Verification items for the finished model (mm, model axes). Face numbers are marked on the shaded views. Round coordinates to 2 decimals unless told otherwise and drop trailing zeros. Loops run counter-clockwise (first coordinate to the right, second up) from the corner with the lowest first, then second, coordinate; pieces in that order, holes last. Notation, with made-up numbers: (-37.75, -6.75) - (13.25, -6.75) arc R16 cw to (13.25, 6.25) - close; hole circle Ø4 at (66.5, -24.5). An arc over 180 degrees is marked (long way). Use CSV: the item, a comma, the result in double quotes.
```python
from build123d import *

# Parameters (mm, degrees)
SKETCH1_R           = 2.637642313
SKETCH1_R_2         = 73
BOSS_EXTRUDE1_DEPTH = 20
SKETCH4_R           = 73
SKETCH4_R_2         = 52.25
BOSS_EXTRUDE2_DEPTH = 10
SKETCH5_R           = 73
BOSS_EXTRUDE3_DEPTH = 10


with BuildPart() as part:
    # Sketch1 → Boss-Extrude1 (new body)
    with BuildSketch(Plane(origin=(0, 0, 0), x_dir=(1, 0, 0), z_dir=(0, 1, 0))):
        with BuildLine():
            Line((77.460838348, -75.098177713), (77.460838348, 74.577424045))
            ThreePointArc((77.460838348, 74.577424045), (76.578174547, 76.708362964), (74.447235628, 77.591026765))
            Line((74.447235628, 77.591026765), (-75.22836613, 77.591026765))
            ThreePointArc((-75.22836613, 77.591026765), (-77.359305049, 76.708362964), (-78.24196885, 74.577424045))
            Line((-78.24196885, 74.577424045), (-78.24196885, -75.098177713))
            ThreePointArc((-78.24196885, -75.098177713), (-77.359305049, -77.229116632), (-75.22836613, -78.111780433))
            Line((-75.22836613, -78.111780433), (74.447235628, -78.111780433))
            ThreePointArc((74.447235628, -78.111780433), (76.578174547, -77.229116632), (77.460838348, -75.098177713))
        make_face()
        with Locations((-60.604326536, -60.47413812)):
            Circle(SKETCH1_R, mode=Mode.SUBTRACT)
        with Locations((-60.604326536, 59.953384452)):
            Circle(SKETCH1_R, mode=Mode.SUBTRACT)
        with Locations((59.823196035, 59.953384452)):
            Circle(SKETCH1_R, mode=Mode.SUBTRACT)
        with Locations((59.823196035, -60.47413812)):
            Circle(SKETCH1_R, mode=Mode.SUBTRACT)
        Circle(SKETCH1_R_2, mode=Mode.SUBTRACT)
    extrude(amount=BOSS_EXTRUDE1_DEPTH)

    # Sketch4 → Boss-Extrude2 (add)
    with BuildSketch(Plane(origin=(0, 20, 0), x_dir=(1, 0, 0), z_dir=(0, 1, 0))):
        Circle(SKETCH4_R)
        Circle(SKETCH4_R_2, mode=Mode.SUBTRACT)
    extrude(amount=-BOSS_EXTRUDE2_DEPTH)

    # Sketch5 → Boss-Extrude3 (add)
    with BuildSketch(Plane.XZ.offset(-10)):
        Circle(SKETCH5_R)
    extrude(amount=BOSS_EXTRUDE3_DEPTH)


solid = part.part
```
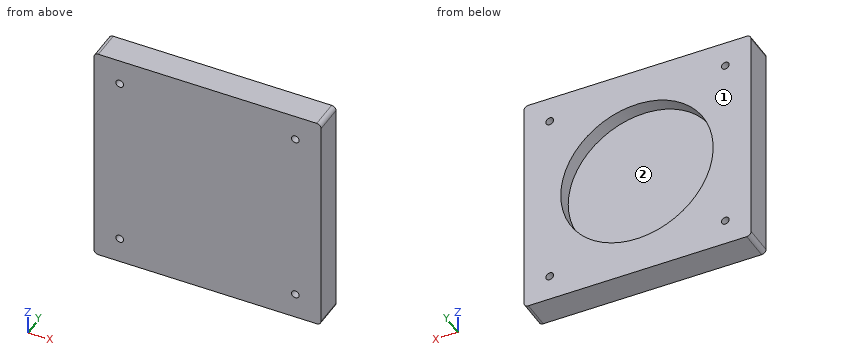
1) Thickness scan on probe 1 along X at (y, z) = (10.75, 0.5); probe 2 along Z at (x, y) = (0, 16.75); probe 3 along Z at (x, y) = (60.5, 18). Record the ranges inside material, lowest first. Write a range as [from, to].
Returned:
probe 1,"x = [-78.24, -52.25], [52.25, 77.46]"
probe 2,"z = [-77.59, -52.25], [52.25, 78.11]"
probe 3,"z = [-77.59, -62.5], [-57.4, 57.92], [63.02, 78.11]"
2) Cross-section at C-C, the plane y = 13.75. Record the cut outline in (x, z), then the cut area to 3 significant figures.
Returned:
outline,"(-78.24, -74.58) arc R3.01 ccw to (-75.23, -77.59) - (74.45, -77.59) arc R3.01 ccw to (77.46, -74.58) - (77.46, 75.1) arc R3.01 ccw to (74.45, 78.11) - (-75.23, 78.11) arc R3.01 ccw to (-78.24, 75.1) - close; hole circle Ø5.28 at (-60.6, -59.95); hole circle Ø5.28 at (-60.6, 60.47); hole circle Ø104.5 at (0, 0); hole circle Ø5.28 at (59.82, -59.95); hole circle Ø5.28 at (59.82, 60.47)"
area,"15,600 mm²"
3) Mould release check, pull along X, two halves, no side actions. Record for the marked faces 1 and 2: +X half, -X half, draft (parallel to the pull), parting line (faces both ways), or undercut.
Returned:
face 1,"draft"
face 2,"undercut"
4) Cross-section at B-B, the plane z = 0. Record the cut outline in (x, y).
Returned:
outline,"(-78.24, 0) - (77.46, 0) - (77.46, 20) - (52.25, 20) - (52.25, 10) - (-52.25, 10) - (-52.25, 20) - (-78.24, 20) - close"
5) Gauge pin test, flat end, axial feed: pin 1 Ø3 at (x, z) = (-60.6, 60.47) entering from +Y. Record the tip position at first contact, or that the pin passes through.
Returned:
pin 1,"passes through"
6) Cross-section at A-A, the plane x = 0. Record the cut outline in (y, z), then the cut area to 3 significant figures.
Returned:
outline,"(0, -77.59) - (20, -77.59) - (20, -52.25) - (10, -52.25) - (10, 52.25) - (20, 52.25) - (20, 78.11) - (0, 78.11) - close"
area,"2,070 mm²"
